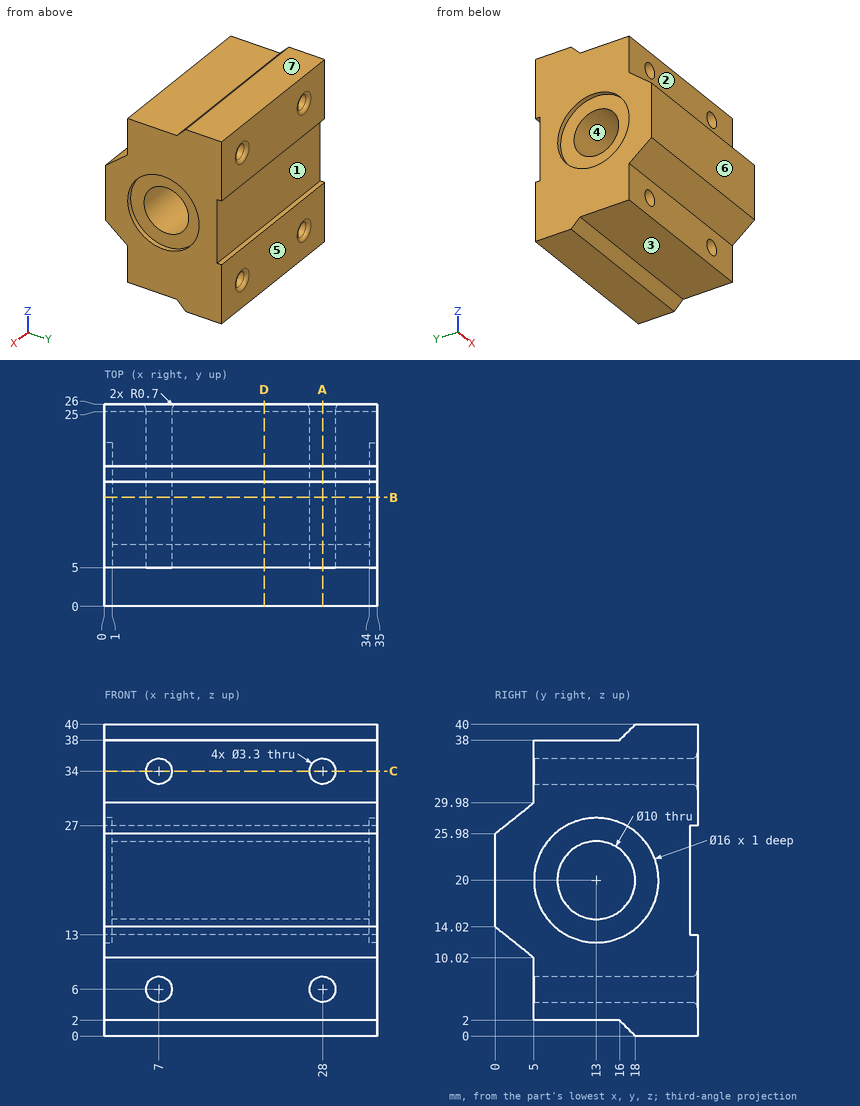
Check sheet for the drawn part. Datum: minimum x, y, z corner. Units: mm. A direction names the side the tool comes from. Round coordinates to 2 decimals unless told otherwise and drop trailing zeros. Loops run counter-clockwise (first coordinate to the right, second up) from the corner with the lowest first, then second, coordinate; pieces in that order, holes last.
Item 1: Cross-section at C-C on z = 34. Record the boundary of the cut face in (x, y).
Item 2: Thickness scan on line 1 (X direction, y = 18.75, z = 34); line 2 (Z direction, x = 29.5, y = 18.25); line 3 (Z direction, x = 7, y = 12.75). Record the ranges inside material, lowest first.
Item 3: Access from +Z, -Z, +X, -X, +Y, -Y to the whole of each face (thin tool, end or side, straight path). Record for the marked faces 1, 2 and 3.
Item 4: Gauge pin test, flat ends, axial feed: pin 1 (4 mm diameter, centred on x = 7, z = 34, fed in from -Y); pin 2 (10 mm diameter, centred on x = 19.5, y = 3.5, fed in from -Z); pin 3 (8 mm diameter, centred on x = 5.5, z = 16.5, fed in from +Y); pin 4 (4 mm diameter, centred on x = 30, y = 10.5, fed in from +Z). Record the tip position at first contact, or that the pin passes through.
Item 5: Cross-section at B-B on y = 14. Record the boundary of the cut face in (x, z), then the cut area to 3 significant figures.
Item 6: Mould release check, pull along Y, two halves, no side actions. Record for the marked faces 4, 5, 6 and 7: pulls with the +Y half, pulls with the -Y half, needs draft (parallel to the pull), parting line crosses it, or undercut.
Item 7: Cross-section at D-D on x = 20.5. Record the boundary of the cut face in (y, z).
Item 8: Cross-section at A-A on x = 28. Count the separate pieces of the cut face and the enclosed holes in it, then the cut area to 3 significant figures.
Answer sheet:
1. outline: (0, 5) - (5.35, 5) - (5.35, 25.3) arc R0.7 ccw to (4.65, 26) - (0, 26) - close; (8.65, 5) - (26.35, 5) - (26.35, 25.3) arc R0.7 ccw to (25.65, 26) - (9.35, 26) arc R0.7 ccw to (8.65, 25.3) - close; (29.65, 5) - (35, 5) - (35, 26) - (30.35, 26) arc R0.7 ccw to (29.65, 25.3) - close
2. line 1: x = 0 to 5.35, 8.65 to 26.35, 29.65 to 35
2. line 2: z = 0 to 5.31, 6.69 to 33.31, 34.69 to 40
2. line 3: z = 2 to 4.35, 7.65 to 15.01, 24.99 to 32.35, 35.65 to 38
3. face 1: +X, -X, +Y
3. face 2: +Z, +X, -X, -Y
3. face 3: -Z, +X, -X, -Y
4. pin 1: stops at y = 5
4. pin 2: stops at z = 2
4. pin 3: stops at y = 26
4. pin 4: stops at z = 38
5. outline: (0, 2) - (35, 2) - (35, 12.06) - (34, 12.06) - (34, 15.1) - (1, 15.1) - (1, 12.06) - (0, 12.06) - close; (0, 27.94) - (1, 27.94) - (1, 24.9) - (34, 24.9) - (34, 27.94) - (35, 27.94) - (35, 38) - (0, 38) - close; hole circle Ø3.3 at (7, 6); hole circle Ø3.3 at (7, 34); hole circle Ø3.3 at (28, 6); hole circle Ø3.3 at (28, 34)
5. area: 871 mm2
6. face 4: undercut
6. face 5: pulls with the +Y half
6. face 6: pulls with the -Y half
6. face 7: needs draft
7. outline: (0, 14.02) - (5, 10.02) - (5, 2) - (16, 2) - (18, 0) - (26, 0) - (26, 13) - (25, 13) - (25, 27) - (26, 27) - (26, 40) - (18, 40) - (16, 38) - (5, 38) - (5, 29.98) - (0, 25.98) - close; hole circle Ø10 at (13, 20)
8. separate pieces: 3
8. enclosed holes: 1
8. area: 640 mm2
